from build123d import *

# Parameters (mm, degrees)
F1_DEPTH = 2082.8
F3_DEPTH = 152.4
F5_DEPTH = 152.4


with BuildPart() as f1:
    # F0 (on Front) → F1 (new body)
    with BuildSketch(Plane.XZ):
        with BuildLine():
            Line((0, 152.4), (0, 0))
            Line((0, 0), (20.955, 0))
            Line((20.955, 0), (20.955, 136.525))
            ThreePointArc((20.955, 136.525), (17.14516, 145.595503), (8.001, 149.225))
            Line((8.001, 149.225), (8.001, 152.4))
            Line((8.001, 152.4), (0, 152.4))
        make_face()
    extrude(amount=-F1_DEPTH)

    # F2 (on face) → F3 (cut)
    with BuildSketch(Plane(origin=(0, 0, 0), x_dir=(1, 0, 0), z_dir=(0, 0, -1))):
        Polygon((0, -20.955), (20.955, 0), (0, 0), align=None)
    extrude(amount=-F3_DEPTH, mode=Mode.SUBTRACT)

    # F4 (on face) → F5 (cut)
    with BuildSketch(Plane(origin=(0, 0, 0), x_dir=(1, 0, 0), z_dir=(0, 0, -1))):
        Polygon((0, -2082.8), (20.955, -2082.8), (0, -2061.845), align=None)
    extrude(amount=-F5_DEPTH, mode=Mode.SUBTRACT)


solid = f1.part
Read the model definition and answer for the solid it produces. Units are mm, in the model's axes. Coordinates: 2 decimals unless noted, no trailing zeros. Loops run counter-clockwise (first coordinate to the right, second up) from the corner with the lowest first, then second, coordinate; pieces in that order, holes last.
Q1. Consider probe 1 along Z at (x, y) = (8.5, 516); probe 2 along Y at (x, z) = (8, 90) (3 decimals); probe 3 along Y at (x, z) = (5.75, 55.5) (3 decimals). Determine where each line is inside the solid, lowest interval first.
Q2. The part is cut by section B-B on x = 17.5. Write down the section's boundary in (y, z) (3 decimals).
Q3. The part is cut by section A-A on y = 1634.5. Write down the section's boundary in (x, z) (1 decimal), and give its area (3 significant figures).
Q4. Each of these flat-tipped pins is pushed along its axis until it touches: pin 1 Ø5 at (x, z) = (2.5, 38) entering from +Y (3 decimals); pin 2 Ø6 at (x, z) = (6.5, 135) entering from +Y (3 decimals); pin 3 Ø3 at (x, z) = (6, 43) entering from -Y (3 decimals). Where does it stop, or does it pass through?
Results below:
1. probe 1: z = 0 to 149.23
1. probe 2: y = 12.955 to 2069.845
1. probe 3: y = 15.205 to 2067.595
2. outline: (3.455, 0) - (2079.345, 0) - (2079.345, 145.233) - (3.455, 145.233) - close
3. outline: (0, 0) - (21, 0) - (21, 136.5) arc R12.7 ccw to (8, 149.2) - (8, 152.4) - (0, 152.4) - close
3. area: 3,120 mm2
4. pin 1: stops at y = 2066.845
4. pin 2: stops at y = 2071.345
4. pin 3: stops at y = 13.455
